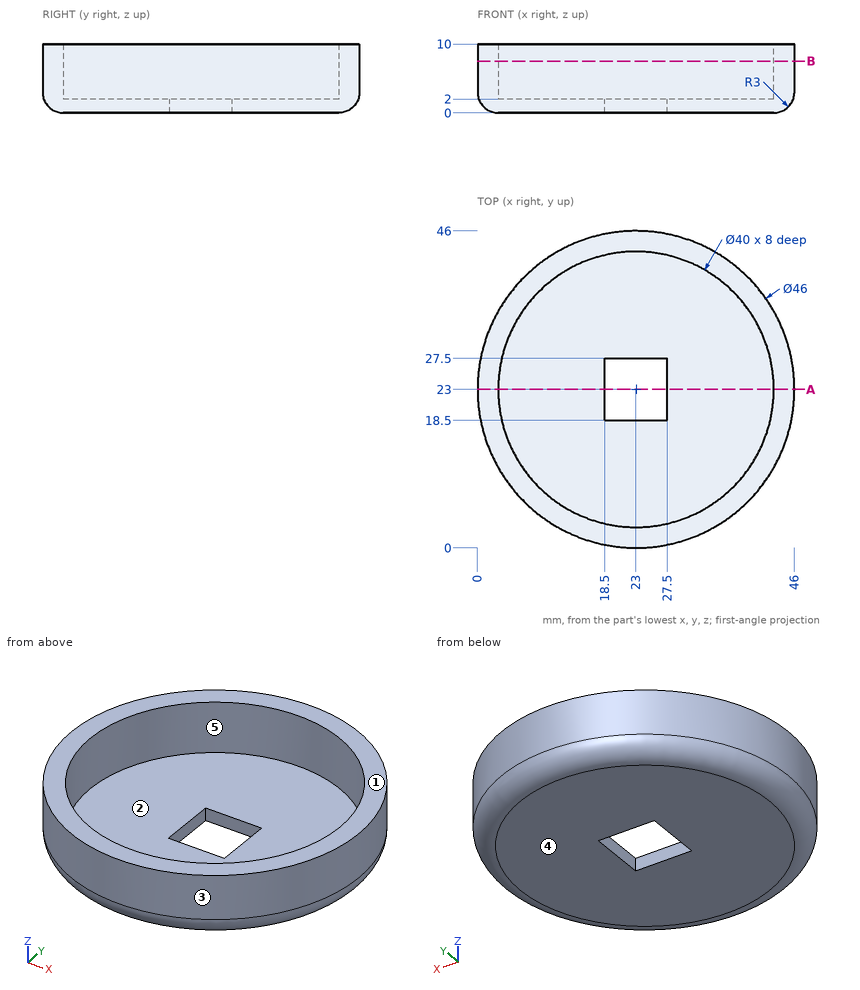
The figure shows three views and two pictorial views of one solid part (mm, origin at its lowest corner). Answer the questions. A direction names the side the tool comes from. Give positions to 0.01 mm unless a question says otherwise; leave off trailing zeros. Order: outer loops, then holes, each group sorted by start corner. A loop starts at its lowest first (then second) coordinate and runs counter-clockwise, first axis right, second up. Notation, with made-up numbers: (84.25, 64) -> (136.25, 64) arc R20 ccw to (136.25, 79) -> close; hole circle Ø10 at (57.5, -2). An arc over 180 degrees is marked (long way). Answer as a JSON object with one key per item and string values. Group by question number.
Item 1: The part is cut by section B-B on z = 7.5. Write down the section's boundary in (x, y), and give its area (3 significant figures).
Item 2: Determine the mould class of the marked faces 1, 2 and 3 for opening direction X: pulls with the +X half, pulls with the -X half, needs draft (parallel to the pull), parting line crosses it, or undercut.
Item 3: The part is cut by section A-A on y = 23. Write down the section's boundary in (x, z), and give its area (3 significant figures).
Item 4: Flat-ended cylindrical pins translate along their axes: pin 1 (20 mm diameter, centred on x = 28, y = 20, fed in from +Z); pin 2 (3 mm diameter, centred on y = 40, z = 3.5, fed in from +X); pin 3 (0.6 mm diameter, centred on x = 23.5, z = 1, fed in from +Y). Find the tip coordinate at first contact, or state that the pin passes through.
Item 5: A tool of negligible diameter and unlimited length cuts with its end or side. For the marked faces 4 and 5, from which of +Z, -Z, +X, -X, +Y, -Y can it reach the whole face along a straight path? Write none if from no direction.
Item 6: Consider L1, parallel to Y at x = 23, z = 7.25; L2, parallel to Y at x = 9.5, z = 7; L3, parallel to Z at x = 32.5, y = 27. Determine where each line is inside the solid, lowest interval first. Write a range as from..to.
Result set:
{
 "1": {"outline": "circle Ø46 at (23, 23); hole circle Ø40 at (23, 23)", "area": "405 mm²"},
 "2": {"face 1": "needs draft", "face 2": "undercut", "face 3": "parting line crosses it"},
 "3": {"outline": "(0, 3) arc R3 ccw to (3, 0) -> (18.5, 0) -> (18.5, 2) -> (3, 2) -> (3, 10) -> (0, 10) -> close; (27.5, 0) -> (43, 0) arc R3 ccw to (46, 3) -> (46, 10) -> (43, 10) -> (43, 2) -> (27.5, 2) -> close", "area": "118 mm²"},
 "4": {"pin 1": "z = 2", "pin 2": "x = 39.99", "pin 3": "y = 45.47"},
 "5": {"face 4": "-Z, +X, -X, +Y, -Y", "face 5": "+Z"},
 "6": {"L1": "0..3, 43..46", "L2": "4.38..8.24, 37.76..41.62", "L3": "0..2"}
}
